Part print with two shaded views. Sizes in mm from the minimum x, y, z corner. A direction names the side the tool comes from. Give positions to 0.01 mm unless a question says otherwise; leave off trailing zeros. Write each loop counter-clockwise with the first axis right and the second up, starting at its lowest first coordinate (ties: lowest second). Pieces come first, ordered by that corner, then holes.
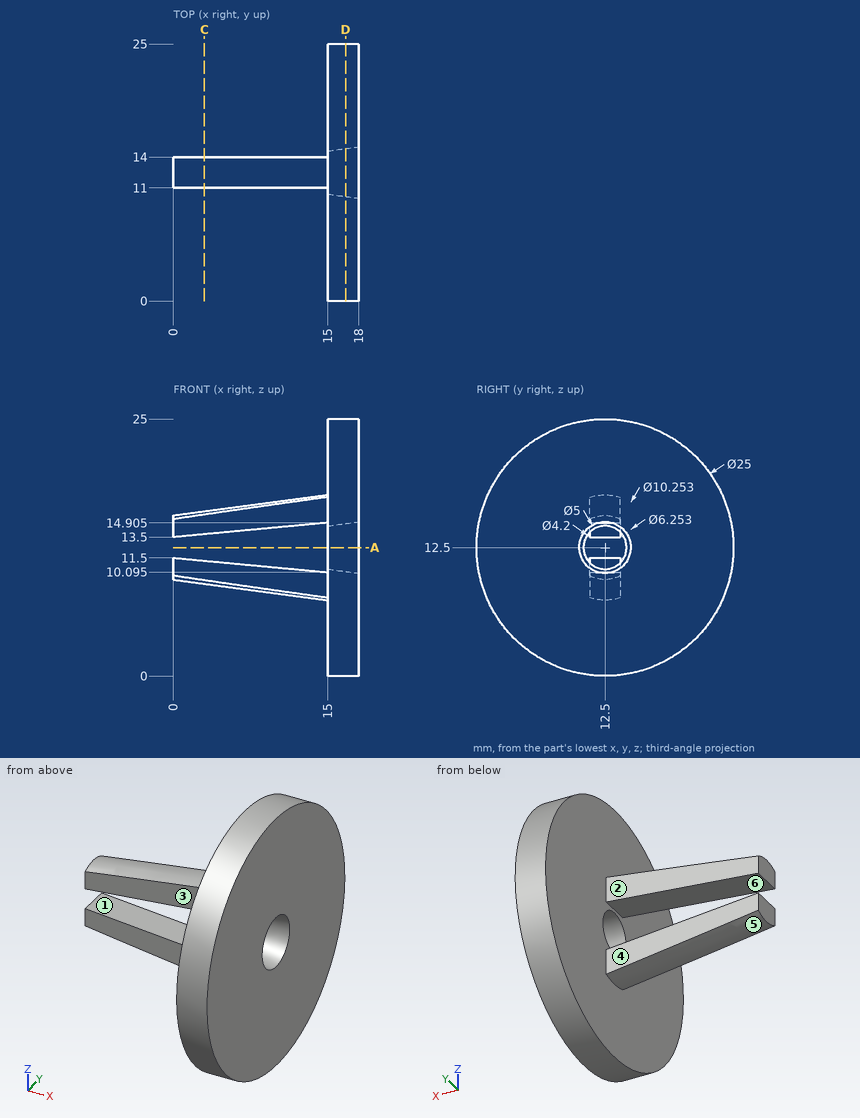
(1) Saw through at A-A, the plane z = 12.5. List the corners of the cut face in (x, y).
(2) Saw through at C-C, the plane x = 3. List the corners of the cut face in (y, z), plus the area to 3 significant figures.
(3) 3-axis set-ups, long thin cutter, end or side, ignore diameter. For the marked faces 1, 2 and 3: which of +Z, -Z, +X, -X, +Y, -Y reach the whole face in a straight line?
(4) Drop flat-ended pins along their axis: pin 1 (6 mm diameter, centred on x = 16, y = 21, fed in from +Z) (1 decimal); pin 2 (6 mm diameter, centred on x = 14, z = 17.5, fed in from -Y); pin 3 (3 mm diameter, centred on x = 9.5, z = 10.5, fed in from +Y). Give the stop position or say it passes through.
(5) Saw through at D-D, the plane x = 16.75. List the corners of the cut face in (y, z).
(6) Mould opens along Z. For the marked faces 4, 5 and 6 say: +Z half, -Z half, draft (parallel to the pull), parting line (faces both ways), or undercut.
(7) Probe line 1 (X direction, y = 16.5, z = 3.75); line 2 (Y direction, x = 13.25, z = 8.5); line 3 (Z direction, x = 6.75, y = 12.5). List the from-to ranges inside material, lowest first.
Computed values:
1. outline: (15, 0) - (18, 0) - (18, 10) - (15, 10.4) - close; (15, 14.6) - (18, 15) - (18, 25) - (15, 25) - close
2. outline: (11, 9.31) arc R3.53 ccw to (14, 9.31) - (14, 11.22) - (11, 11.22) - close; (11, 13.78) - (14, 13.78) - (14, 15.69) arc R3.53 ccw to (11, 15.69) - close
2. area: 12.8 mm2
3. face 1: +Y, -Y
3. face 2: +Z, -Z, -X, +Y
3. face 3: +Z, -Z, -X, -Y
4. pin 1: stops at z = 23.7
4. pin 2: stops at y = 0.19
4. pin 3: stops at y = 14
5. outline: circle Ø25 at (12.5, 12.5); hole circle Ø4.67 at (12.5, 12.5)
6. face 4: draft
6. face 5: -Z half
6. face 6: undercut
7. line 1: x = 15 to 18
7. line 2: y = 11 to 14
7. line 3: z = 8.47 to 10.87, 14.13 to 16.53
